Autodesk Inventor part; units mm, degrees
ref_plane "additional_rod_XY" through (0, 0, 0) normal (0, 1, 0) x (1, 0, 0)
ref_plane "additional_rod_YZ" through (0, 0, 0) normal (1, 0, 0) x (0, 0, -1)
ref_plane "additional_rod_ZX" through (0, 0, 0) normal (0, 0, -1) x (0, 1, 0)
sketch "Sketch_1" plane through (0, 0, 0) normal (0, 0, 1) x (1, 0, 0)
  line L0 (0, 0) -> (0, 52.832)
  line L1 (0, 52.832) -> (3.048, 52.832)
  line L2 (3.048, 52.832) -> (3.048, 0)
  line L3 (3.048, 0) -> (0, 0)
  line L4 (0, 0) -> (0, 52.832)
revolve "Revolution1" add sketch "Sketch_1" angle 360 about axis through (0, 0, 0) along (0, -1, 0)
sketch "Sketch_3" plane through (0, 0, 0) normal (0, 0, 1) x (1, 0, 0)
  line L0 (0, 0) -> (0, 2.54)
  line L1 (1.524, 0) -> (3.048, 0)
  line L2 (3.048, 0) -> (3.048, 2.54)
  line L3 (3.048, 2.54) -> (1.524, 2.54)
  line L4 (1.524, 2.54) -> (1.524, 0)
revolve "Revolution2" cut sketch "Sketch_3" angle 360 about axis through (0, 0, 0) along (0, -1, 0)
sketch "Sketch_4" plane through (0, 0, 0) normal (0, 0, 1) x (1, 0, 0)
  line L0 (0, 50.292) -> (0, 52.832)
  line L1 (1.524, 52.832) -> (1.524, 50.292)
  line L2 (1.524, 50.292) -> (3.048, 50.292)
  line L3 (3.048, 50.292) -> (3.048, 52.832)
  line L4 (3.048, 52.832) -> (1.524, 52.832)
revolve "Revolution3" cut sketch "Sketch_4" angle 360 about axis through (0, 50.292, 0) along (0, -1, 0)
ref_plane "additional_rod_XY" through (0, 0, 0) normal (0, 1, 0) x (1, 0, 0)
ref_plane "additional_rod_YZ" through (0, 0, 0) normal (1, 0, 0) x (0, 0, -1)
ref_plane "additional_rod_ZX" through (0, 0, 0) normal (0, 0, -1) x (0, 1, 0)
properties part number "022.08-FO1_BM_r" material "Steel"
Read the model definition and answer for the solid it produces. Units are mm, in the model's axes. A direction names the side the tool comes from. Give positions to 0.01 mm unless a question says otherwise; leave off trailing zeros. Write each loop counter-clockwise with the first axis right and the second up, starting at its lowest first coordinate (ties: lowest second). Pieces come first, ordered by that corner, then holes. Notation, with made-up numbers: (4, -32.75) -> (28, -32.75) arc R24 cw to (28, 0.25) -> close; hole circle Ø6 at (53.5, 5.25). An arc over 180 degrees is marked (long way). Answer as a JSON object with one key per item and string values. Group by question number.
1) Each of these flat-tipped pins is pushed along its axis until it touches: P1, Ø1, axis at x = -0.5, y = 38.5, coming from the +Z side; P2, Ø3, axis at y = 25.5, z = 2.5, coming from the -X side; P3, Ø2, axis at x = 2, z = -2, coming from the -Y side. Where does it stop, or does it pass through?
2) A tool of negligible diameter and unlimited length cuts with its end or side. For faces 1 (the flat face through (1.3, 2.54, -1.3)), 2 (the flat face through (0, 0, 0)), 3 (the cylindrical face through (-0.2, 51.54, 1.51)), from which of +Z, -Z, +X, -X, +Y, -Y can it reach the whole face along a straight path? Write none if from no direction.
3) Find section A-A (x = 0). Write down the section's boundary in (y, z).
4) Find section D-D (z = -2). Write down the section's boundary in (x, y), and give its area (3 significant figures).
5) Find section C-C (y = 39.5). Write down the section's boundary in (x, z).
6) Consider L1, parallel to Y at x = 1, z = 1.25; L2, parallel to X at y = 46.5, z = 0.25; L3, parallel to X at y = 5, z = 2. Determine where each line is inside the solid, lowest interval first. Write a range as from..to.
7) Find section B-B (z = 0). Write down the section's boundary in (x, y).
8) The mould has two halves that part along Z. Classify faces 4 (the cylindrical face through (-0.4, 26.08, 3.02)), 5 (the flat face through (1.3, 50.292, -1.3)): +Z half, -Z half, draft (parallel to the pull), parting line (faces both ways), or undercut.
Values follow:
{
 "1": {"P1": "stops at z = 3.05", "P2": "stops at x = -2.88", "P3": "stops at y = 2.54"},
 "2": {"face 1": "-Y", "face 2": "+Z, -Z, +X, -X, -Y", "face 3": "+Y"},
 "3": {"outline": "(0, -1.52) -> (2.54, -1.52) -> (2.54, -3.05) -> (50.29, -3.05) -> (50.29, -1.52) -> (52.83, -1.52) -> (52.83, 1.52) -> (50.29, 1.52) -> (50.29, 3.05) -> (2.54, 3.05) -> (2.54, 1.52) -> (0, 1.52) -> close"},
 "4": {"outline": "(-2.3, 2.54) -> (2.3, 2.54) -> (2.3, 50.29) -> (-2.3, 50.29) -> close", "area": "220 mm2"},
 "5": {"outline": "circle Ø6.1 at (0, 0)"},
 "6": {"L1": "y = 2.54..50.29", "L2": "x = -3.04..3.04", "L3": "x = -2.3..2.3"},
 "7": {"outline": "(-3.05, 2.54) -> (-1.52, 2.54) -> (-1.52, 0) -> (1.52, 0) -> (1.52, 2.54) -> (3.05, 2.54) -> (3.05, 50.29) -> (1.52, 50.29) -> (1.52, 52.83) -> (-1.52, 52.83) -> (-1.52, 50.29) -> (-3.05, 50.29) -> close"},
 "8": {"face 4": "parting line", "face 5": "draft"}
}
